from build123d import *

# Parameters (mm, degrees)
F0_R     = 15.875
F2_DEPTH = 6.35
F3_D     = 3.175
F4_R     = 5.08


with BuildPart() as f2:
    # F0 (on Front) → F2 (new body)
    with BuildSketch(Plane.XZ):
        Circle(F0_R)
    extrude(amount=F2_DEPTH)

    # F3 (through all)
    with Locations(Plane(origin=(0, 0, 0), x_dir=(1, 0, 0), z_dir=(0, 1, 0))):
        with Locations((3.9598953958, -2.8153994276), (-3.3950347352, -2.5255896296), (-3.5310642417, 4.9982398479), (3.925069736, 4.9148391505)):
            Hole(F3_D / 2)

    # F4
    f4_edges = [f2.edges().sort_by_distance(p)[0] for p in [
        (-15.875, -6.35, 0),
    ]]
    fillet(f4_edges, radius=F4_R)


solid = f2.part
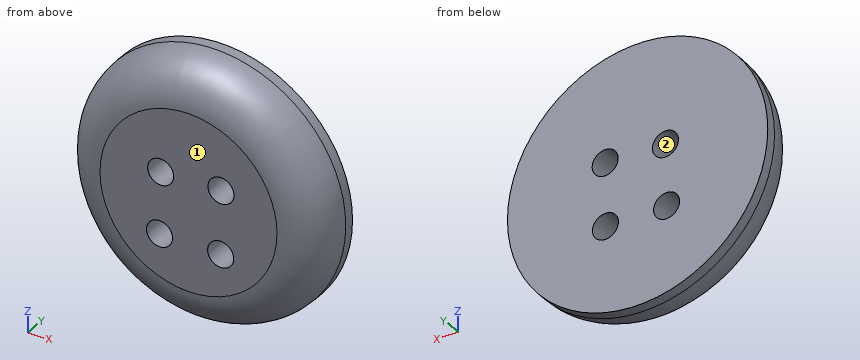
Geometry check sheet. Reference: the model listing, model coordinates, mm. Face numbers are marked on the shaded views. Give positions to 0.01 mm unless a question says otherwise; leave off trailing zeros. Write each loop counter-clockwise with the first axis right and the second up, starting at its lowest first coordinate (ties: lowest second). Pieces come first, ordered by that corner, then holes. Notation, with made-up numbers: M -35,-12 L 19,-12 A8 cw 19,-7 Z; hole C -14,48 d11. An arc over 180 degrees is marked long. One line per question, with ' | ' between items.
1. Cross-section at D-D (y = -2). Enter the section's corners in (x, z) (1 decimal), plus the area to 3 significant figures.
Ans:
outline: C 0,0 d31.6; hole C -3.5,-5 d3.2; hole C -3.4,2.5 d3.2; hole C 3.9,-4.9 d3.2; hole C 4,2.8 d3.2 | area: 755 mm2
2. Cross-section at A-A (y = -3.75). Enter the section's corners in (x, z) (1 decimal), plus the area to 3 significant figures.
Ans:
outline: C 0,0 d30.5; hole C -3.5,-5 d3.2; hole C -3.4,2.5 d3.2; hole C 3.9,-4.9 d3.2; hole C 4,2.8 d3.2 | area: 697 mm2
3. Gauge pin test, flat ends, axial feed: pin 1 (3 mm diameter, centred on y = -1.5, z = -3, fed in from +X); pin 2 (1 mm diameter, centred on y = -5, z = 9.5, fed in from -X); pin 3 (1.5 mm diameter, centred on y = -5.5, z = -1, fed in from -X). Record the tip position at first contact, or that the pin passes through.
Ans:
pin 1: x = 15.8 | pin 2: x = -11.38 | pin 3: x = -14.46
4. Mould release check, pull along X, two halves, no side actions. Record for the marked faces 1 and 2: released by +X, released by -X, zero draft, split by the parting line, or undercut.
Ans:
face 1: zero draft | face 2: undercut
5. Cross-section at C-C (x = 0). Enter the section's corners in (y, z) (3 decimals).
Ans:
outline: M -6.35,-10.795 A5.08 ccw -1.27,-15.875 L 0,-15.875 L 0,15.875 L -1.27,15.875 A5.08 ccw -6.35,10.795 Z
6. Cross-section at B-B (z = 0). Enter the section's corners in (x, y) (3 decimals).
Ans:
outline: M -15.875,-1.27 A5.08 ccw -10.795,-6.35 L 10.795,-6.35 A5.08 ccw 15.875,-1.27 L 15.875,0 L -15.875,0 Z
7. Scan lines: line 1 along Z through (x, y) = (-4.5, -1); line 2 along X through (y, z) = (-4.5, -4); line 3 along X through (y, z) = (-5.5, 1.5). Record each from-to range of solid material in increasing order. Write a range as from..to.
Ans:
line 1: -15.22..-6.26, -3.74..1.39, 3.67..15.22 | line 2: -14.16..-4.77, -2.3..2.63, 5.22..14.16 | line 3: -13.53..-4.61, -2.18..3.07, 4.85..13.53
